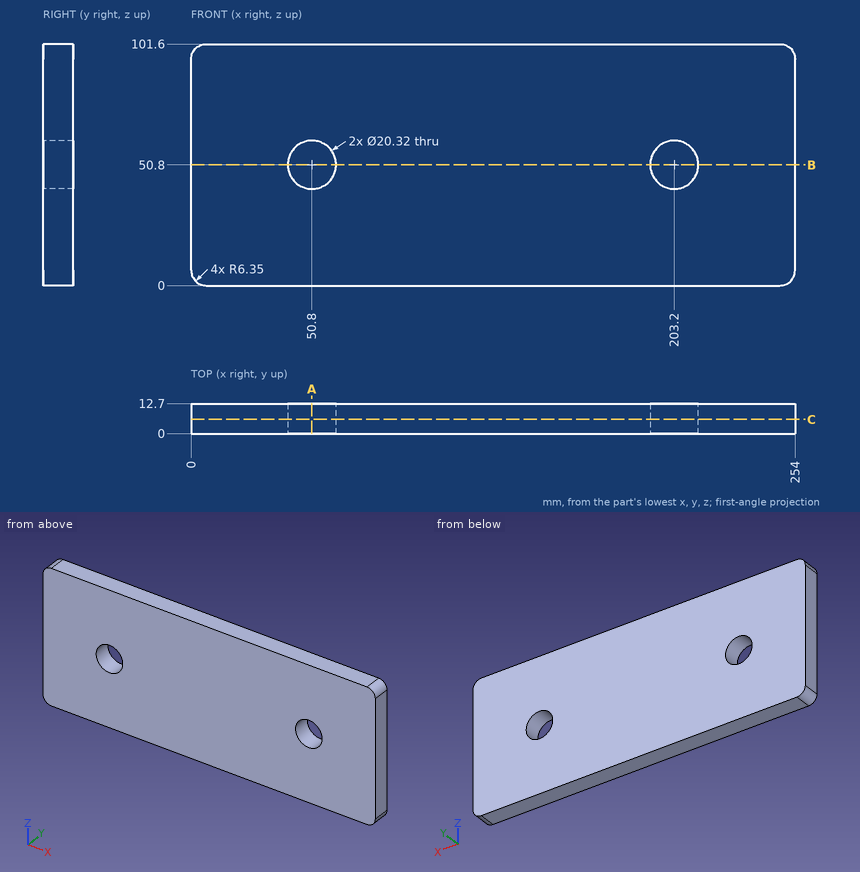
Answer from the drawing. Dimensions are ordinates in mm from the lowest x, y and z of the part. Round coordinates to 2 decimals unless told otherwise and drop trailing zeros. Write each loop counter-clockwise with the first axis right and the second up, starting at its lowest first coordinate (ties: lowest second). Pieces come first, ordered by that corner, then holes. Notation, with made-up numbers: M -33,74 L 9,74 A15 ccw 9,79 Z; hole C 32,78.5 d3. An arc over 180 degrees is marked long. Write each question's results on one line, items separated by ' | '. Start each with the question number.
Item 1: A cutting plane is placed at A-A on x = 50.8. Write down the section's boundary in (y, z), and give its area (3 significant figures).
Item 2: A cutting plane is placed at B-B on z = 50.8. Write down the section's boundary in (x, y), and give its area (3 significant figures).
Item 3: Straight lines are drawn through the part: L1, parallel to Z at x = 50.8, y = 3.25; L2, parallel to X at y = 2.5, z = 50.5. For each, find the intervals that lie inside material, in ascending order. Write a range as [from, to].
Item 4: A cutting plane is placed at C-C on y = 6. Write down the section's boundary in (x, z).
Item 5: A flat-ended cylindrical pin translates along its axis: pin 1 Ø2 at (x, z) = (208.5, 45.5) entering from -Y. Find the tip coordinate at first contact, or state that the pin passes through.
Check sheet entries:
1) outline: M 0,0 L 12.7,0 L 12.7,40.64 L 0,40.64 Z; M 0,60.96 L 12.7,60.96 L 12.7,101.6 L 0,101.6 Z | area: 1,030 mm²
2) outline: M 0,0 L 40.64,0 L 40.64,12.7 L 0,12.7 Z; M 60.96,0 L 193.04,0 L 193.04,12.7 L 60.96,12.7 Z; M 213.36,0 L 254,0 L 254,12.7 L 213.36,12.7 Z | area: 2,710 mm²
3) L1: [0, 40.64], [60.96, 101.6] | L2: [0, 40.64], [60.96, 193.04], [213.36, 254]
4) outline: M 0,6.35 A6.35 ccw 6.35,0 L 247.65,0 A6.35 ccw 254,6.35 L 254,95.25 A6.35 ccw 247.65,101.6 L 6.35,101.6 A6.35 ccw 0,95.25 Z; hole C 50.8,50.8 d20.32; hole C 203.2,50.8 d20.32
5) pin 1: through
